from build123d import *
from build123d.topology import SkipClean

# Parameters (mm, degrees)
SKETCH1_W           = 21
SKETCH1_H           = 21
BOSS_EXTRUDE1_DEPTH = 10.5
CUT_EXTRUDE1_DEPTH  = 24.5
CUT_EXTRUDE2_DEPTH  = 24.5
CUT_EXTRUDE3_DEPTH  = 24.5
SKETCH5_R           = 16.5
BOSS_EXTRUDE2_DEPTH = 17
CHAMFER4_SIZE       = 3
CHAMFER5_SIZE       = 3
SKETCH13_R          = 10
BOSS_EXTRUDE6_DEPTH = 5
SKETCH14_R          = 2.5
CUT_EXTRUDE7_DEPTH  = 10


with BuildPart() as part:
    # Sketch1 → Boss-Extrude1 (new body)
    with BuildSketch(Plane(origin=(0, 0, 0), x_dir=(1, 0, 0), z_dir=(0, 1, 0))):
        with Locations((1.107272727, 1.909090909)):
            Rectangle(SKETCH1_W, SKETCH1_H)
    extrude(amount=BOSS_EXTRUDE1_DEPTH)

    # Sketch2 → Cut-Extrude1 (cut)
    with BuildSketch(Plane.XY.offset(8.590909091)):
        with BuildLine():
            ThreePointArc((3.607272727, 5.25), (2.87503968, 7.017766953), (1.107272727, 7.75))
            Line((1.107272727, 7.75), (1.107272727, 2.75))
            ThreePointArc((1.107272727, 2.75), (2.87503968, 3.482233047), (3.607272727, 5.25))
        make_face()
        with BuildLine():
            Line((1.107272727, 2.75), (1.107272727, 7.75))
            ThreePointArc((1.107272727, 7.75), (-1.392727273, 5.25), (1.107272727, 2.75))
        make_face()
    extrude(amount=-CUT_EXTRUDE1_DEPTH, mode=Mode.SUBTRACT)

    # Sketch3 → Cut-Extrude2 (cut)
    with BuildSketch(Plane.ZY.offset(9.392727273)):
        with BuildLine():
            ThreePointArc((0.590909091, 5.25), (-0.141323956, 7.017766953), (-1.909090909, 7.75))
            Line((-1.909090909, 7.75), (-1.909090909, 2.75))
            ThreePointArc((-1.909090909, 2.75), (-0.141323956, 3.482233047), (0.590909091, 5.25))
        make_face()
        with BuildLine():
            Line((-1.909090909, 2.75), (-1.909090909, 7.75))
            ThreePointArc((-1.909090909, 7.75), (-4.409090909, 5.25), (-1.909090909, 2.75))
        make_face()
    extrude(amount=-CUT_EXTRUDE2_DEPTH, mode=Mode.SUBTRACT)

    # Sketch4 → Cut-Extrude3 (cut)
    with SkipClean():  # the faces are left unmerged after this step: merging them gives an invalid solid
        with BuildSketch(Plane(origin=(0, 10.5, 0), x_dir=(1, 0, 0), z_dir=(0, 1, 0))):
            with BuildLine():
                ThreePointArc((-9.392727273, 1.909090919), (-6.317348472, 9.333712115), (1.107272727, 12.409090909))
                Line((1.107272727, 12.409090909), (-9.392727273, 12.409090909))
                Line((-9.392727273, 12.409090909), (-9.392727273, 1.909090919))
            make_face()
            with BuildLine():
                Line((11.607272727, 12.409090909), (1.107272727, 12.409090909))
                ThreePointArc((1.107272727, 12.409090909), (8.53189393, 9.333712112), (11.607272727, 1.909090909))
                Line((11.607272727, 1.909090909), (11.607272727, 12.409090909))
            make_face()
            with BuildLine():
                ThreePointArc((11.607272727, 1.909090909), (8.53189393, -5.515530293), (1.107272727, -8.590909091))
                Line((1.107272727, -8.590909091), (11.607272727, -8.590909091))
                Line((11.607272727, -8.590909091), (11.607272727, 1.909090909))
            make_face()
            with BuildLine():
                Line((-9.392727273, -8.590909091), (1.107272727, -8.590909091))
                ThreePointArc((1.107272727, -8.590909091), (-6.317348479, -5.51553029), (-9.392727273, 1.909090919))
                Line((-9.392727273, 1.909090919), (-9.392727273, -8.590909091))
            make_face()
        extrude(amount=-CUT_EXTRUDE3_DEPTH, mode=Mode.SUBTRACT)

    # Sketch5 → Boss-Extrude2 (add)
    with SkipClean():  # the faces are left unmerged after this step: merging them gives an invalid solid
        with BuildSketch(Plane(origin=(0, 10.5, 0), x_dir=(1, 0, 0), z_dir=(0, 1, 0))):
            with Locations(Location((1.107272727, 1.909090909, 0), (0, 0, 270))):
                Circle(SKETCH5_R)
        extrude(amount=BOSS_EXTRUDE2_DEPTH)

    # Chamfer4
    chamfer4_edges = [part.edges().sort_by_distance(p)[0] for p in [
        (1.107272727, 27.5, -18.409090909),
    ]]
    chamfer(chamfer4_edges, length=CHAMFER4_SIZE)

    # Chamfer5
    chamfer5_edges = [part.edges().sort_by_distance(p)[0] for p in [
        (1.107272727, 10.5, -18.409090909),
    ]]
    chamfer(chamfer5_edges, length=CHAMFER5_SIZE)

    # Sketch13 → Boss-Extrude6 (add)
    with SkipClean():  # the faces are left unmerged after this step: merging them gives an invalid solid
        with BuildSketch(Plane.XZ):
            with Locations(Location((1.107272727, -1.909090909, 0), (0, 0, 270))):
                Circle(SKETCH13_R)
        extrude(amount=BOSS_EXTRUDE6_DEPTH)

    # Sketch14 → Cut-Extrude7 (cut)
    with SkipClean():  # the faces are left unmerged after this step: merging them gives an invalid solid
        with BuildSketch(Plane.XZ.offset(5)):
            with Locations(Location((1.107272727, -1.909090909, 0), (0, 0, 270))):
                Circle(SKETCH14_R)
        extrude(amount=-CUT_EXTRUDE7_DEPTH, mode=Mode.SUBTRACT)


solid = part.part
The model under review builds one solid part; all positions refer to its coordinate system, in mm. A direction names the side the tool comes from. Round coordinates to 2 decimals unless told otherwise and drop trailing zeros. Write each loop counter-clockwise with the first axis right and the second up, starting at its lowest first coordinate (ties: lowest second). Pieces come first, ordered by that corner, then holes. Notation, with made-up numbers: (31.5, 83.25) -> (77.5, 83.25) arc R30 cw to (77.5, 114.25) -> close; hole circle Ø5 at (24, 45.25). An arc over 180 degrees is marked (long way). Answer as a JSON object with one key per item and string values.
1. To check wall thickness, follow line 1 along Z through (x, y) = (1, 21.5); line 2 along Y through (x, z) = (9, 5.5); line 3 along Y through (x, z) = (-6, 5.5). State the ranges of each line that lie inside material, in increasing order.
Results found:
{"line 1": "z = -18.41 to 14.59", "line 2": "y = 10.5 to 27.5", "line 3": "y = 0 to 27.5"}
2. We need section B-B on y = -2.5. State the section outline as (x, z) points.
Results found:
{"outline": "circle Ø20 at (1.11, -1.91); hole circle Ø5 at (1.11, -1.91)"}
3. We need section A-A on y = 8.5. State the section outline as (x, z) points.
Results found:
{"outline": "circle Ø21 at (1.11, -1.91)"}
4. We need section C-C on z = -2.5. State how many separate pieces and enclosed holes the cut face has, and give its area (3 significant figures).
Results found:
{"separate pieces": "3", "enclosed holes": "0", "area": "723 mm^2"}
5. The part is to be moulded in two halves that separate along X. For faces 1 (the face through (1, 27.5, -2)), 2 (the face through (-12.214, 10.646, -4.867)), 3 (the face through (1.22, -0.82, 0.59)), say which applies: pulls with the +X half, pulls with the -X half, needs draft (parallel to the pull), parting line crosses it, or undercut.
Results found:
{"face 1": "needs draft", "face 2": "parting line crosses it", "face 3": "undercut"}
6. Clearance check with flat-ended pins moving along their axes: pin 1 (8 mm diameter, centred on x = 13, z = 9.5, fed in from +Y); pin 2 (4 mm diameter, centred on x = -5.5, y = 22, fed in from -Z); pin 3 (2 mm diameter, centred on y = 3.5, z = 0.5, fed in from +X); pin 4 (8 mm diameter, centred on x = 3.5, y = -1, fed in from +Z). State where each tip first meets the part, or that it passes through.
Results found:
{"pin 1": "stops at y = 27.5", "pin 2": "stops at z = -17.75", "pin 3": "stops at x = 11.51", "pin 4": "stops at z = 8.59"}
7. Machinability: for faces 4 (the face through (-1, -5, -4)), 5 (the face through (11.022, -2.465, -0.607)), which of the approach directions +Z, -Z, +X, -X, +Y, -Y give a long, thin tool a straight path to every point of the face, cutting with its end or side? Answer none if there is none.
Results found:
{"face 4": "+Z, -Z, +X, -X, -Y", "face 5": "-Y"}
8. We need section D-D on y = 22. State the section outline as (x, z) points.
Results found:
{"outline": "circle Ø33 at (1.11, -1.91)"}
